Source: CAD feature listing. Evaluate the final solid. Frame: model axes, mm. Face numbers are marked on the shaded views. Give positions to 0.01 mm unless a question says otherwise; leave off trailing zeros. Loops run counter-clockwise (first coordinate to the right, second up) from the corner with the lowest first, then second, coordinate; pieces in that order, holes last.
Autodesk Inventor part; units mm, degrees
ref_plane "YZ Plane" through (0, 0, 0) normal (1, 0, 0) x (0, 1, 0)
ref_plane "XZ Plane" through (0, 0, 0) normal (0, 1, 0) x (-1, 0, 0)
ref_plane "XY Plane" through (0, 0, 0) normal (0, 0, 1) x (1, 0, 0)
sketch "Эскиз1" plane through (0, 0, 0) normal (0, 0, 1) x (1, 0, 0)
  circle A0 centre (0, 0) radius 4
  circle A1 centre (0, 0) radius 6.5
extrude "Выдавливание1" add sketch "Эскиз1" along normal blind 1
sketch "Эскиз2" plane through (0, 0, 1) normal (0, 0, 1) x (1, 0, 0)
  circle A0 centre (0, 0) radius 4
  circle A1 centre (0, 0) radius 6.5
  circle A2 centre (0, 0) radius 6
  circle A3 centre (0, 0) radius 4.5
  dimension "d2" = 12
  dimension "d3" = 9
extrude "Выдавливание2" add sketch "Эскиз2" along normal blind 0.7
properties part number "Cap"
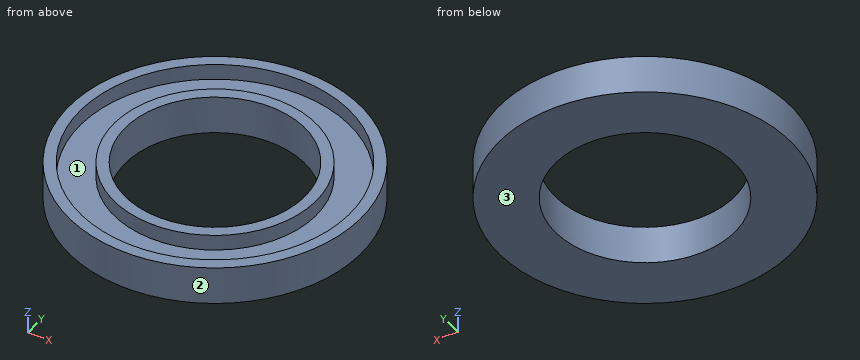
1) Cut plane A-A (z = 1.3). Return loops of the section in (x, y), and give its area (3 significant figures).
Checks:
outline: circle Ø13 at (0, 0); circle Ø9 at (0, 0); hole circle Ø12 at (0, 0); hole circle Ø8 at (0, 0)
area: 33.0 mm2
2) Pull-direction query (X, two-part tool) for the marked faces 1, 2 and 3; classes: released by +X, released by -X, zero draft, split by the parting line, or undercut.
Checks:
face 1: undercut
face 2: split by the parting line
face 3: zero draft
3) Contact query for a flat-ended pin moving along its axis: P1, Ø1, axis at y = 4.5, z = 1, coming from the +X side. Output: stop coordinate, or through.
Checks:
P1: stops at x = 5.12
4) Cut plane C-C (x = -1). Return loops of the section in (y, z).
Checks:
outline: (-6.42, 0) - (-3.87, 0) - (-3.87, 1.7) - (-4.39, 1.7) - (-4.39, 1) - (-5.92, 1) - (-5.92, 1.7) - (-6.42, 1.7) - close; (3.87, 0) - (6.42, 0) - (6.42, 1.7) - (5.92, 1.7) - (5.92, 1) - (4.39, 1) - (4.39, 1.7) - (3.87, 1.7) - close
5) Cut plane B-B (y = 0). Return loops of the section in (x, z).
Checks:
outline: (-6.5, 0) - (-4, 0) - (-4, 1.7) - (-4.5, 1.7) - (-4.5, 1) - (-6, 1) - (-6, 1.7) - (-6.5, 1.7) - close; (4, 0) - (6.5, 0) - (6.5, 1.7) - (6, 1.7) - (6, 1) - (4.5, 1) - (4.5, 1.7) - (4, 1.7) - close
6) Ray query, probe 1 along Y at (x, z) = (0, 1.55); probe 2 along Y at (x, z) = (0, 0.75); probe 3 along X at (y, z) = (-2.75, 1.3). Return the intervals inside material, ascending.
Checks:
probe 1: y = -6.5 to -6, -4.5 to -4, 4 to 4.5, 6 to 6.5
probe 2: y = -6.5 to -4, 4 to 6.5
probe 3: x = -5.89 to -5.33, -3.56 to -2.9, 2.9 to 3.56, 5.33 to 5.89
7) Cut plane D-D (x = 4.75). Return loops of the section in (y, z).
Checks:
outline: (-4.44, 0) - (4.44, 0) - (4.44, 1.7) - (3.67, 1.7) - (3.67, 1) - (-3.67, 1) - (-3.67, 1.7) - (-4.44, 1.7) - close
